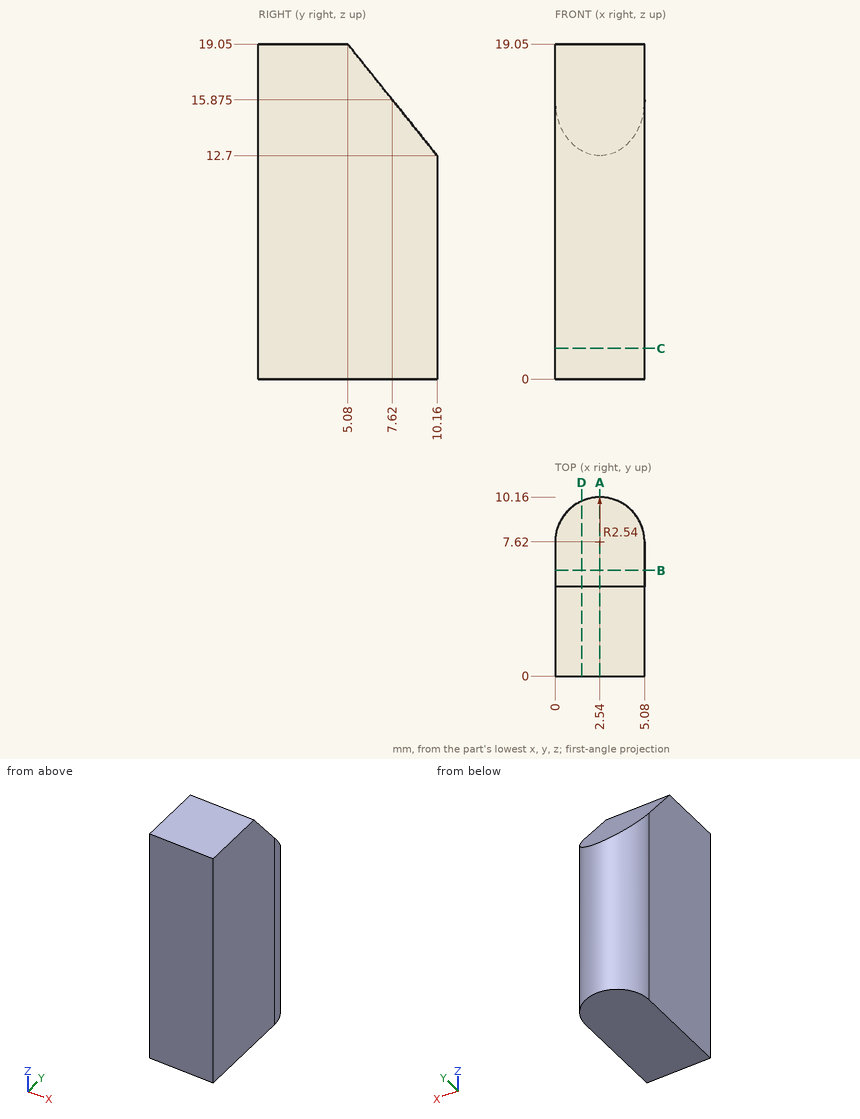
The drawing under review shows one solid part. Ordinate dimensions are in mm from its lowest x, y, z. Give positions to 0.01 mm unless a question says otherwise; leave off trailing zeros. Order: outer loops, then holes, each group sorted by start corner. A loop starts at its lowest first (then second) coordinate and runs counter-clockwise, first axis right, second up. Notation, with made-up numbers: M -25,-24 L 28,-24 A19 cw 28,-15 Z; hole C 88.5,-4 d4. An arc over 180 degrees is marked long. Answer in a Markdown table with one row per item. Add a question column.
1. To check wall thickness, follow line 1 along X through (y, z) = (7.75, 12.25); line 2 along Y through (x, z) = (2.45, 8); line 3 along X through (y, z) = (8.5, 4.5). State the ranges of each line that lie inside material, in increasing order.
2. Add section C-C on z = 1.75. State the section outline as (x, y) points.
3. Add section A-A on x = 2.54. State the section outline as (y, z) points, plus the area to 3 significant figures.
4. For pin 1 Ø5 at (y, z) = (8, 11) entering from +X; pin 2 Ø2 at (x, z) = (1.5, 15.5) entering from +Y, all flat-tipped, find the tip position at first contact; note any pin that passes through.
5. Add section B-B on y = 6. State the section outline as (x, z) points.
6. Add section D-D on x = 1.5. State the section outline as (y, z) points.
The answers:
| question | item | result |
|---|---|---|
| 1 | line 1 | 0 to 5.08 |
| 1 | line 2 | 0 to 10.16 |
| 1 | line 3 | 0.16 to 4.92 |
| 2 | outline | M 0,0 L 5.08,0 L 5.08,7.62 A2.54 ccw 0,7.62 Z |
| 3 | outline | M 0,0 L 10.16,0 L 10.16,12.7 L 5.08,19.05 L 0,19.05 Z |
| 3 | area | 177 mm2 |
| 4 | pin 1 | x = 5.08 |
| 4 | pin 2 | y = 8.72 |
| 5 | outline | M 0,0 L 5.08,0 L 5.08,17.9 L 0,17.9 Z |
| 6 | outline | M 0,0 L 9.94,0 L 9.94,12.98 L 5.08,19.05 L 0,19.05 Z |
